from build123d import *

# Parameters (mm, degrees)
F_01_HOUSING_PROFILE_W        = 210
F_01_HOUSING_PROFILE_H        = 190
F_01_HOUSING_PROFILE_R        = 8
F_01_HOUSING_BLOCK_DEPTH      = 220
F_02_FACE_BOSS_PROFILE_R      = 72.5
F_02_FACE_LOCATING_BOSS_DEPTH = 245
F_03_OUTPUT_SHAFT_PROFILE_R   = 30
F_03_OUTPUT_SHAFT_DEPTH       = 285


with BuildPart() as part:
    # 01_Housing_Profile → 01_Housing_Block (new body)
    with BuildSketch(Plane(origin=(0, 0, 0), x_dir=(1, 0, 0), z_dir=(0, 1, 0))):
        Rectangle(F_01_HOUSING_PROFILE_W, F_01_HOUSING_PROFILE_H)
        with Locations(Location((66.519326341, 27.55320713, 0), (0, 0, 270))):
            Circle(F_01_HOUSING_PROFILE_R, mode=Mode.SUBTRACT)
        with Locations(Location((27.55320713, 66.519326341, 0), (0, 0, 270))):
            Circle(F_01_HOUSING_PROFILE_R, mode=Mode.SUBTRACT)
        with Locations(Location((-27.55320713, 66.519326341, 0), (0, 0, 270))):
            Circle(F_01_HOUSING_PROFILE_R, mode=Mode.SUBTRACT)
        with Locations(Location((-66.519326341, 27.55320713, 0), (0, 0, 270))):
            Circle(F_01_HOUSING_PROFILE_R, mode=Mode.SUBTRACT)
        with Locations(Location((-66.519326341, -27.55320713, 0), (0, 0, 270))):
            Circle(F_01_HOUSING_PROFILE_R, mode=Mode.SUBTRACT)
        with Locations(Location((-27.55320713, -66.519326341, 0), (0, 0, 270))):
            Circle(F_01_HOUSING_PROFILE_R, mode=Mode.SUBTRACT)
        with Locations(Location((27.55320713, -66.519326341, 0), (0, 0, 270))):
            Circle(F_01_HOUSING_PROFILE_R, mode=Mode.SUBTRACT)
        with Locations(Location((66.519326341, -27.55320713, 0), (0, 0, 270))):
            Circle(F_01_HOUSING_PROFILE_R, mode=Mode.SUBTRACT)
    extrude(amount=F_01_HOUSING_BLOCK_DEPTH)

    # 02_Face_Boss_Profile → 02_Face_Locating_Boss (add)
    with BuildSketch(Plane(origin=(0, 0, 0), x_dir=(1, 0, 0), z_dir=(0, 1, 0))):
        with Locations(Location((0, 0, 0), (0, 0, 73.835030621))):
            Circle(F_02_FACE_BOSS_PROFILE_R)
    extrude(amount=F_02_FACE_LOCATING_BOSS_DEPTH)

    # 03_Output_Shaft_Profile → 03_Output_Shaft (add)
    with BuildSketch(Plane(origin=(0, 0, 0), x_dir=(1, 0, 0), z_dir=(0, 1, 0))):
        with Locations(Location((0, 0, 0), (0, 0, 270))):
            Circle(F_03_OUTPUT_SHAFT_PROFILE_R)
    extrude(amount=F_03_OUTPUT_SHAFT_DEPTH)


solid = part.part
Part model, mm, in its own coordinate system. A direction names the side the tool comes from. Coordinates: 2 decimals unless noted, no trailing zeros. Loops run counter-clockwise (first coordinate to the right, second up) from the corner with the lowest first, then second, coordinate; pieces in that order, holes last. Notation, with made-up numbers: (47, 1) -> (79, 1) arc R20 ccw to (79, 25) -> close; hole circle Ø9 at (49.25, 29). An arc over 180 degrees is marked (long way). Use a Markdown table: item, result. Add a question column.
Item 1: Band-saw the part on C-C on y = 73.5. Give the number of separate pieces and of enclosed holes in the cut face, plus the area to 3 significant figures.
Item 2: Flat gauge pins, fed straight in: P1, Ø2, axis at x = 37.5, z = 15, coming from the +Y side; P2, Ø12, axis at x = -56, z = -66, coming from the +Y side. Where does each tip first touch, or does it go through?
Item 3: Band-saw the part on D-D on z = 43.5. Write the cut outline in (x, y), plus the area to 3 significant figures.
Item 4: Which spindle directions (+Z, -Z, +X, -X, +Y, -Y) get a long thin tool onto all of the face, cutting with end or side? Do faces 1 (the flat face through (0, 285, 0)), 2 (the flat face through (8, 245, -30)). Say none if no direction does.
Item 5: Band-saw the part on A-A on z = 0. Write the cut outline in (x, y), plus the area to 3 significant figures.
Item 6: Probe probe 1 along X at (y, z) = (115.5, -24); probe 2 along Z at (x, y) = (32, 205.5); probe 3 along Z at (x, y) = (31, 99). List the from-to ranges inside material, lowest first.
Item 7: Pull direction Z, two halves, no side cores. Call faces 3 (the cylindrical face through (1.32, 264.72, -29.97)), 4 (the cylindrical face through (-73.84, 108.46, -30.78)), 5 (the flat face through (-71, 220, 20)): +Z half, -Z half, draft (parallel to the pull), parting line (faces both ways), or undercut.
Item 8: Band-saw the part on B-B on x = 0. Write the cut outline in (y, z), plus the area to 3 significant figures.
Geometry says:
| question | item | result |
|---|---|---|
| 1 | separate pieces | 1 |
| 1 | enclosed holes | 8 |
| 1 | area | 39,100 mm² |
| 2 | P1 | y = 245 |
| 2 | P2 | y = 220 |
| 3 | outline | (-105, 0) -> (105, 0) -> (105, 220) -> (58, 220) -> (58, 245) -> (-58, 245) -> (-58, 220) -> (-105, 220) -> close |
| 3 | area | 49,100 mm² |
| 4 | face 1 | +Z, -Z, +X, -X, +Y |
| 4 | face 2 | +Y |
| 5 | outline | (-105, 0) -> (105, 0) -> (105, 220) -> (72.5, 220) -> (72.5, 245) -> (30, 245) -> (30, 285) -> (-30, 285) -> (-30, 245) -> (-72.5, 245) -> (-72.5, 220) -> (-105, 220) -> close |
| 5 | area | 52,200 mm² |
| 6 | probe 1 | -105 to -73.69, -68.41 to 68.41, 73.69 to 105 |
| 6 | probe 2 | -95 to -73.17, -65.06 to 65.06, 73.17 to 95 |
| 6 | probe 3 | -95 to -73.74, -65.54 to 65.54, 73.74 to 95 |
| 7 | face 3 | parting line |
| 7 | face 4 | undercut |
| 7 | face 5 | draft |
| 8 | outline | (0, -95) -> (220, -95) -> (220, -72.5) -> (245, -72.5) -> (245, -30) -> (285, -30) -> (285, 30) -> (245, 30) -> (245, 72.5) -> (220, 72.5) -> (220, 95) -> (0, 95) -> close |
| 8 | area | 47,800 mm² |
